from build123d import *

# Parameters (mm, degrees)
SWEEP1_START             = -29.3624001
SWEEP1_OUTLINE_R         = 2.1844
SWEEP1_DEPTH             = 29.3624001
SWEEP1_2_OUTLINE_R       = 2.1844
SWEEP1_2_ANGLE           = 180
SWEEP1_3_OUTLINE_R       = 2.1844
SWEEP1_3_ANGLE           = 180
BOSS_EXTRUDE1_DEPTH      = 0.254
BOSS_EXTRUDE1_DEPTH_BACK = 19.1262


with BuildPart() as part:
    # Sweep1: read off the stored shape, not the designer's step
    # Sweep1 outline → Sweep1 (new body)
    with BuildSketch(Plane.XY.offset(SWEEP1_START)):
        with Locations((8.5344, 0)):
            Circle(SWEEP1_OUTLINE_R)
        with Locations((-8.5344, 0)):
            Circle(SWEEP1_OUTLINE_R)
    extrude(amount=SWEEP1_DEPTH)

    # Sweep1 2 outline → Sweep1 2 (revolve)
    with BuildSketch(Plane.XY.offset(-29.3624)):
        with Locations((8.5344, 0)):
            Circle(SWEEP1_2_OUTLINE_R)
    revolve(axis=Axis((0, 0, -29.3624), (0, 1, 0)), revolution_arc=SWEEP1_2_ANGLE)

    # Sweep1 3 outline → Sweep1 3 (revolve)
    with BuildSketch(Plane(origin=(0, 0, 0), x_dir=(-1, 0, 0), z_dir=(0, 0, -1))):
        with Locations((8.5344, 0)):
            Circle(SWEEP1_3_OUTLINE_R)
    revolve(axis=Axis((0, 0, 0), (0, 1, 0)), revolution_arc=SWEEP1_3_ANGLE)

    # Sketch2 → Boss-Extrude1 (add, two sides: drawn at the far end of the back side and taken through both)
    with BuildSketch(Plane.XY.offset(-BOSS_EXTRUDE1_DEPTH_BACK)):
        Polygon((13.12445011, 0), (10.829425055, 3.9751), (6.239374945, 3.9751), (3.94434989, 0), (6.239374945, -3.9751), (10.829425055, -3.9751), align=None)
    extrude(amount=BOSS_EXTRUDE1_DEPTH + BOSS_EXTRUDE1_DEPTH_BACK)


solid = part.part
Check sheet for the modelled part. Datum: model origin and axes. Units: mm. A direction names the side the tool comes from. Round coordinates to 2 decimals unless told otherwise and drop trailing zeros. Order: outer loops, then holes, each group sorted by start corner. A loop starts at its lowest first (then second) coordinate and runs counter-clockwise, first axis right, second up. Notation, with made-up numbers: M 15.25,-3 L 25.25,-3 A6 cw 25.25,6 Z; hole C 18,88 d10. An arc over 180 degrees is marked long. One line per item, written item: value. Start each with the question number.
1. Gauge pin test, flat ends, axial feed: P1, Ø10, axis at x = 1.5, z = -2.5, coming from the +Y side; P2, Ø4, axis at x = 11, y = -0.5, coming from the -Z side; P3, Ø2, axis at x = 7.5, y = 2, coming from the -Z side; P4, Ø1, axis at x = -8, y = 2, coming from the -Z side. Record the tip position at first contact, or that the pin passes through.
2. Section check A-A on z = -17.5. Enter the section's corners in (x, y), and give its area (3 significant figures).
3. Release check for a two-part mould opening along X. For faces 1 (the flat face through (11.96, -2.02, -9.57)), 2 (the flat face through (11, 1, -19.126)), 3 (the flat face through (9, 3.975, -10)) record: released by +X, released by -X, zero draft, split by the parting line, or undercut.
4. Scan lines: line 1 along X through (y, z) = (0, -27.5); line 2 along Z through (x, y) = (6.75, 2.75); line 3 along X through (y, z) = (-1.75, -21). Record each from-to range of solid material in increasing order.
5. Access from +Z, -Z, +X, -X, +Y, -Y to the whole of each face (thin tool, end or side, straight path). Record for faces 4 (the cylindrical face through (6.352, 0.096, -24.316)), 5 (the flat face through (5.1, -2, -9.6)), 6 (the flat face through (5.1, 2, -9.6)).
Results found:
1. P1: y = 3.98
1. P2: z = -35.13
1. P3: z = -37.1
1. P4: z = -35.78
2. outline: C -8.53,0 d4.37; M 3.94,0 L 6.24,-3.98 L 10.83,-3.98 L 13.12,0 L 10.83,3.98 L 6.24,3.98 Z
2. area: 69.7 mm^2
3. face 1: released by +X
3. face 2: undercut
3. face 3: zero draft
4. line 1: -10.72 to -6.35, 6.35 to 10.72
4. line 2: -19.13 to 0.25
4. line 3: -9.84 to -7.23, 7.23 to 9.84
5. face 4: none
5. face 5: -Y
5. face 6: +Y
